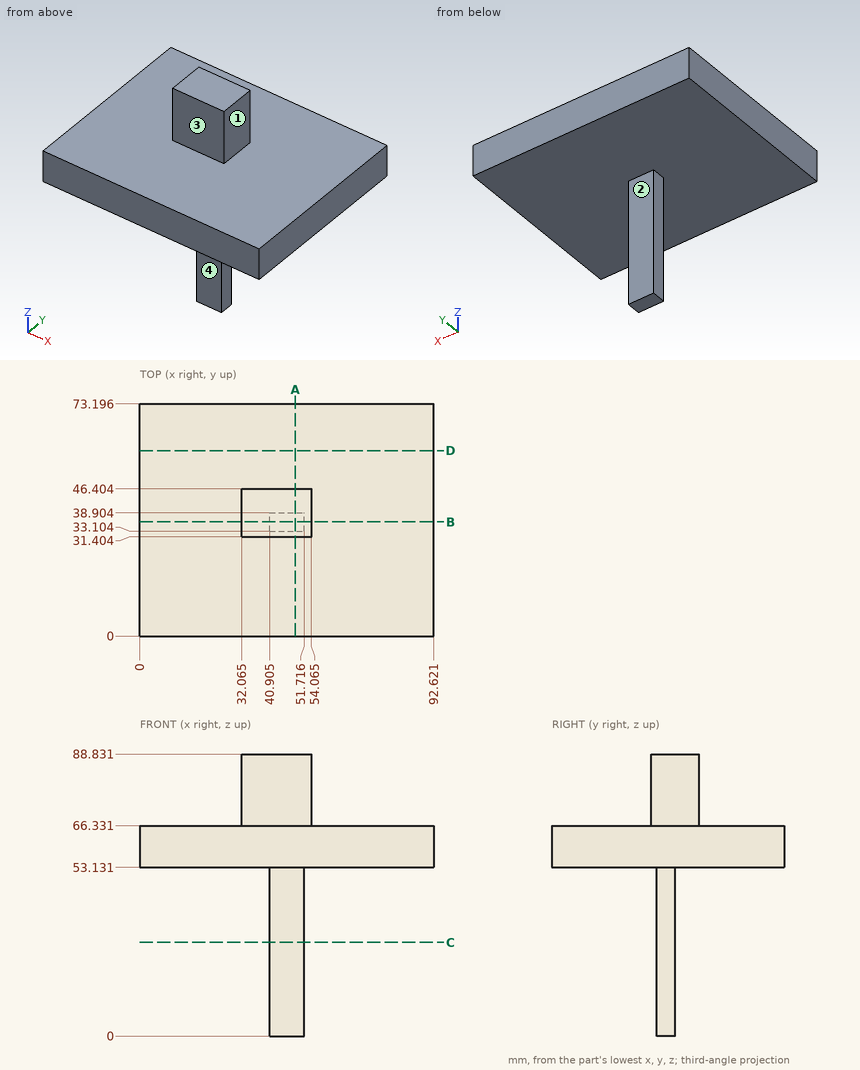
Geometry check sheet. Reference: drawing and pictorial views, mm from the part's lowest x, y, z. A direction names the side the tool comes from. Coordinates: 2 decimals unless noted, no trailing zeros. Order: outer loops, then holes, each group sorted by start corner. A loop starts at its lowest first (then second) coordinate and runs counter-clockwise, first axis right, second up. Notation, with made-up numbers: M 21,39.5 L 45,39.5 A23 ccw 45,53.5 Z; hole C 80,89.5 d3. An arc over 180 degrees is marked long. Return JSON: item names as keys, results as strings.
1) Thickness scan on L1, parallel to Z at x = 6.5, y = 46; L2, parallel to Z at x = 39.5, y = 43; L3, parallel to Y at x = 52, z = 67. Record the ranges inside material, lowest first. Write a range as [from, to].
Answer list:
{"L1": "[53.13, 66.33]", "L2": "[53.13, 88.83]", "L3": "[31.4, 46.4]"}
2) Access from +Z, -Z, +X, -X, +Y, -Y to the whole of each face (thin tool, end or side, straight path). Record for the marked faces 1, 2, 3 and 4.
Answer list:
{"face 1": "+Z, +X, +Y, -Y", "face 2": "-Z, +X, -X, +Y", "face 3": "+Z, +X, -X, -Y", "face 4": "-Z, +X, -X, -Y"}
3) Cross-section at B-B, the plane y = 36. Record the boundary of the cut face in (x, z) (1 decimal), and give its area (3 significant figures).
Answer list:
{"outline": "M 0,53.1 L 40.9,53.1 L 40.9,0 L 51.7,0 L 51.7,53.1 L 92.6,53.1 L 92.6,66.3 L 54.1,66.3 L 54.1,88.8 L 32.1,88.8 L 32.1,66.3 L 0,66.3 Z", "area": "2,290 mm2"}
4) Cross-section at C-C, the plane z = 29.5. Record the boundary of the cut face in (x, y) (1 decimal), and give its area (3 significant figures).
Answer list:
{"outline": "M 40.9,33.1 L 51.7,33.1 L 51.7,38.9 L 40.9,38.9 Z", "area": "62.7 mm2"}
5) Cross-section at A-A, the plane x = 49. Record the boundary of the cut face in (y, z) (1 decimal), and give its area (3 significant figures).
Answer list:
{"outline": "M 0,53.1 L 33.1,53.1 L 33.1,0 L 38.9,0 L 38.9,53.1 L 73.2,53.1 L 73.2,66.3 L 46.4,66.3 L 46.4,88.8 L 31.4,88.8 L 31.4,66.3 L 0,66.3 Z", "area": "1,610 mm2"}
6) Cross-section at D-D, the plane y = 58.5. Record the boundary of the cut face in (x, z), and give its area (3 significant figures).
Answer list:
{"outline": "M 0,53.13 L 92.62,53.13 L 92.62,66.33 L 0,66.33 Z", "area": "1,220 mm2"}
7) Gauge pin test, flat ends, axial feed: pin 1 (1 mm diameter, centred on x = 34, z = 72.5, fed in from +Y); pin 2 (4 mm diameter, centred on x = 42, y = 46, fed in from -Z); pin 3 (5.5 mm diameter, centred on x = 47.5, z = 33, fed in from +Y). Record the tip position at first contact, or that the pin passes through.
Answer list:
{"pin 1": "y = 46.4", "pin 2": "z = 53.13", "pin 3": "y = 38.9"}
